Here's how the part is built. I have some questions about the finished solid (model axes, mm). Face numbers are marked on the shaded views. A direction names the side the tool comes from. Coordinates: 2 decimals unless noted, no trailing zeros. Loops run counter-clockwise (first coordinate to the right, second up) from the corner with the lowest first, then second, coordinate; pieces in that order, holes last. Notation, with made-up numbers: (42, 75) - (65, 75) arc R11 ccw to (65, 92) - close; hole circle Ø11 at (56, -6). An arc over 180 degrees is marked (long way). Use a Markdown table: item, result.
```python
from build123d import *

# Parameters (mm, degrees)
SKETCH1_W               = 100
SKETCH1_H               = 100
BOSS_EXTRUDE1_DEPTH     = 15
SKETCH2_R               = 4.01
SKETCH2_W               = 43
SKETCH2_H               = 43
CUT_EXTRUDE1_DEPTH      = 9
SKETCH3_W               = 31.126627524
SKETCH3_H               = 9
CUT_EXTRUDE2_DEPTH      = 28.5
SKETCH4_R               = 1.75
CUT_EXTRUDE3_DEPTH      = 6
SKETCH5_R               = 3.75
CUT_EXTRUDE4_DEPTH      = 3
FILLET1_R               = 10
FILLET2_R               = 5
SKETCH6_W               = 10
SKETCH6_H               = 33
BOSS_EXTRUDE2_DEPTH     = 76
CUT_EXTRUDE5_DEPTH      = 132.99715906
CUT_EXTRUDE5_DEPTH_BACK = 132.99715906
SKETCH7_R               = 1.55
FILLET3_R               = 4
FILLET4_START           = 21.5
FILLET4_DEPTH           = 24
FILLET4_START_2         = -16.5
FILLET4_2_DEPTH         = 33
FILLET4_START_3         = -30.5
FILLET4_3_DEPTH         = 80.5
FILLET4_START_4         = 15
FILLET4_4_OUTLINE_R     = 4.01
FILLET4_4_DEPTH         = 14


with BuildPart() as part:
    # Sketch1 → Boss-Extrude1 (new body)
    with BuildSketch(Plane(origin=(0, 0, 0), x_dir=(1, 0, 0), z_dir=(0, 1, 0))):
        Rectangle(SKETCH1_W, SKETCH1_H)
    extrude(amount=BOSS_EXTRUDE1_DEPTH)

    # Sketch2 → Cut-Extrude1 (cut)
    with BuildSketch(Plane(origin=(0, 15, 0), x_dir=(1, 0, 0), z_dir=(0, 1, 0))):
        with Locations(Location((-26.5, 26.5, 0), (0, 0, 270))):
            Circle(SKETCH2_R)
        with Locations(Location((0, -28.5, 0), (0, 0, 270))):
            Circle(SKETCH2_R)
        with Locations(Location((26.5, 26.5, 0), (0, 0, 270))):
            Circle(SKETCH2_R)
        Rectangle(SKETCH2_W, SKETCH2_H)
    extrude(amount=-CUT_EXTRUDE1_DEPTH, mode=Mode.SUBTRACT)

    # Sketch3 → Cut-Extrude2 (cut)
    with BuildSketch(Plane(origin=(0, 0, -50), x_dir=(-1, 0, 0), z_dir=(0, 0, -1))):
        with Locations((0, 10.5)):
            Rectangle(SKETCH3_W, SKETCH3_H)
    extrude(amount=-CUT_EXTRUDE2_DEPTH, mode=Mode.SUBTRACT)

    # Sketch4 → Cut-Extrude3 (cut)
    with BuildSketch(Plane.XZ):
        with Locations(Location((-15.5, 15.5, 0), (0, 0, 270))):
            Circle(SKETCH4_R)
        with Locations(Location((15.5, 15.5, 0), (0, 0, 270))):
            Circle(SKETCH4_R)
        with Locations(Location((15.5, -15.5, 0), (0, 0, 270))):
            Circle(SKETCH4_R)
        with Locations(Location((-15.5, -15.5, 0), (0, 0, 270))):
            Circle(SKETCH4_R)
    extrude(amount=-CUT_EXTRUDE3_DEPTH, mode=Mode.SUBTRACT)

    # Sketch5 → Cut-Extrude4 (cut)
    with BuildSketch(Plane.XZ):
        with Locations(Location((-15.5, 15.5, 0), (0, 0, 270))):
            Circle(SKETCH5_R)
        with Locations(Location((15.5, 15.5, 0), (0, 0, 270))):
            Circle(SKETCH5_R)
        with Locations(Location((-15.5, -15.5, 0), (0, 0, 270))):
            Circle(SKETCH5_R)
        with Locations(Location((15.5, -15.5, 0), (0, 0, 270))):
            Circle(SKETCH5_R)
    extrude(amount=-CUT_EXTRUDE4_DEPTH, mode=Mode.SUBTRACT)

    # Fillet1
    fillet1_edges = [part.edges().sort_by_distance(p)[0] for p in [
        (50, 7.5, 50),
        (-50, 7.5, 50),
        (-50, 7.5, -50),
        (50, 7.5, -50),
    ]]
    fillet(fillet1_edges, radius=FILLET1_R)

    # Fillet2
    fillet2_edges = [part.edges().sort_by_distance(p)[0] for p in [
        (15.563313762, 15, -35.75),
        (-15.563313762, 15, -35.75),
        (15.563313762, 10.5, -50),
        (0, 6, -50),
        (-15.563313762, 10.5, -50),
        (15.563313762, 10.5, -21.5),
        (-15.563313762, 10.5, -21.5),
    ]]
    fillet(fillet2_edges, radius=FILLET2_R)

    # Sketch6 → Boss-Extrude2 (add)
    with BuildSketch(Plane(origin=(0, 15, 0), x_dir=(1, 0, 0), z_dir=(0, 1, 0))):
        with Locations((26.5, 0)):
            Rectangle(SKETCH6_W, SKETCH6_H)
    extrude(amount=BOSS_EXTRUDE2_DEPTH)

    # Sketch7 → Cut-Extrude5 (cut, two sides: drawn at the far end of the back side and taken through both)
    with BuildSketch(Plane(origin=(31.5, 0, 0), x_dir=(0, 0, -1), z_dir=(1, 0, 0)).offset(-CUT_EXTRUDE5_DEPTH_BACK)):
        with Locations((11.1, 88.1)):
            Circle(SKETCH7_R)
        with Locations((-11.1, 77.8)):
            Circle(SKETCH7_R)
    extrude(amount=CUT_EXTRUDE5_DEPTH + CUT_EXTRUDE5_DEPTH_BACK, mode=Mode.SUBTRACT)

    # Fillet3
    fillet3_edges = [part.edges().sort_by_distance(p)[0] for p in [
        (26.5, 91, 16.5),
        (26.5, 91, -16.5),
    ]]
    fillet(fillet3_edges, radius=FILLET3_R)

    # Fillet4: read off the stored shape, not the designer's step
    # Fillet4 outline → Fillet4 (add)
    with BuildSketch(Plane.YZ.offset(FILLET4_START)):
        with BuildLine():
            Line((15, 16.5), (29, 16.5))
            ThreePointArc((29, 16.5), (19.100505063, 20.600505063), (15, 30.5))
            Line((15, 30.5), (15, 16.5))
        make_face()
        with BuildLine():
            Line((29, -16.5), (15, -16.5))
            Line((15, -16.5), (15, -30.5))
            ThreePointArc((15, -30.5), (19.100505063, -20.600505063), (29, -16.5))
        make_face()
    extrude(amount=FILLET4_DEPTH)

    # Fillet4 2 outline → Fillet4 2 (add)
    with BuildSketch(Plane.XY.offset(FILLET4_START_2)):
        with BuildLine():
            ThreePointArc((45.5, 15), (35.600505063, 19.100505063), (31.5, 29))
            Line((31.5, 29), (31.5, 15))
            Line((31.5, 15), (45.5, 15))
        make_face()
    extrude(amount=FILLET4_2_DEPTH)

    # Fillet4 3 outline → Fillet4 3 (cut)
    with BuildSketch(Plane.XY.offset(FILLET4_START_3)):
        with BuildLine():
            Line((31.5, 30), (31.5, 29))
            ThreePointArc((31.5, 29), (35.600505063, 19.100505063), (45.5, 15))
            Line((45.5, 15), (47, 15))
            Line((47, 15), (47, 30))
            Line((47, 30), (31.5, 30))
        make_face()
    extrude(amount=FILLET4_3_DEPTH, mode=Mode.SUBTRACT)

    # Fillet4 4 outline → Fillet4 4 (cut)
    with BuildSketch(Plane(origin=(0, 0, 0), x_dir=(1, 0, 0), z_dir=(0, 1, 0)).offset(FILLET4_START_4)):
        with Locations((26.5, 26.5)):
            Circle(FILLET4_4_OUTLINE_R)
    extrude(amount=FILLET4_4_DEPTH, mode=Mode.SUBTRACT)


solid = part.part
```
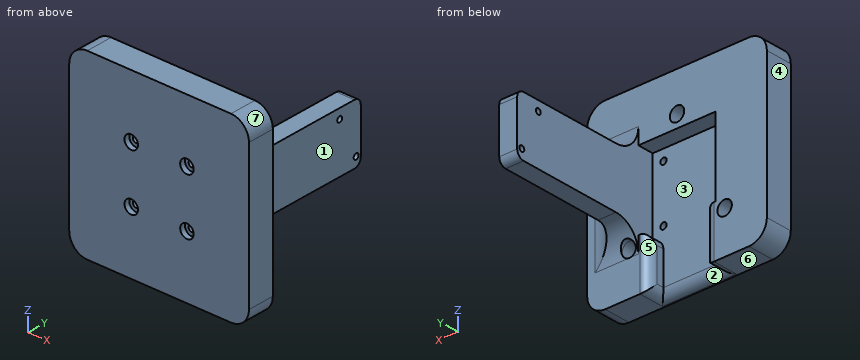
Q1. I want a section at D-D, the plane z = 37.5. Write out the boundary of the cut face in (x, y).
Check values:
| item | result |
|---|---|
| outline | (-50, 0) - (50, 0) - (50, 15) - (-50, 15) - close |
Q2. Will these pins go through, and if not, where does the flat tip stop? P1, Ø8, axis at x = 30.5, y = 54.5, coming from the +Z side; P2, Ø8, axis at x = -19, z = 18.5, coming from the +Y side; P3, Ø10, axis at x = -8.5, z = -18, coming from the +Y side.
Check values:
| item | result |
|---|---|
| P1 | z = 16.5 |
| P2 | y = 15 |
| P3 | y = 6 |
Q3. I want a section at A-A, the plane y = 77.8. Write out the boundary of the cut face in (x, z), then the cut area to 3 significant figures.
Check values:
| item | result |
|---|---|
| outline | (21.5, -16.5) - (31.5, -16.5) - (31.5, 9.55) - (21.5, 9.55) - close; (21.5, 12.65) - (31.5, 12.65) - (31.5, 16.5) - (21.5, 16.5) - close |
| area | 299 mm^2 |
Q4. If we mould it in two halves opening along X, with no side actions, what happens to the marked faces 4, 5, 6 and 7? For each: pulls with the +X half, pulls with the -X half, needs draft (parallel to the pull), parting line crosses it, or undercut.
Check values:
| item | result |
|---|---|
| face 4 | pulls with the -X half |
| face 5 | undercut |
| face 6 | needs draft |
| face 7 | pulls with the +X half |
Q5. Please list where these lines run through material, in increasing order: L1, parallel to X at y = 4.1, z = 15.5; L2, parallel to X at y = 10, z = -26; L3, parallel to X at y = 1.35, z = 15.5. Write a range as from..to.
Check values:
| item | result |
|---|---|
| L1 | -50..-17.25, -13.75..13.75, 17.25..50 |
| L2 | -50..-30.48, -22.52..-15.59, 15.59..22.52, 30.48..50 |
| L3 | -50..-19.25, -11.75..11.75, 19.25..50 |
Q6. Which directions (+Z, -Z, +X, -X, +Y, -Y) give clear straight access to the entire face, cutting with the end or side of a thin tool? Please do the marked faces 1, 2 and 3.
Check values:
| item | result |
|---|---|
| face 1 | +Z, -Z, +X, +Y |
| face 2 | -Z, +Y |
| face 3 | +Y |
Q7. I want a section at B-B, the plane x = 7.5. Write out the boundary of the cut face in (y, z).
Check values:
| item | result |
|---|---|
| outline | (0, -50) - (1, -50) arc R5 ccw to (6, -45) - (6, 21.5) - (15, 21.5) - (15, 50) - (0, 50) - close |
Q8. I want a section at C-C, the plane y = 63.5. Write out the boundary of the cut face in (x, z).
Check values:
| item | result |
|---|---|
| outline | (21.5, -16.5) - (31.5, -16.5) - (31.5, 16.5) - (21.5, 16.5) - close |
